```python
from build123d import *

# Parameters (mm, degrees)
BOSS_EXTRUDE1_DEPTH = 2
FILLET1_R           = 2


with BuildPart() as part:
    # Sketch1 → Boss-Extrude1 (new body)
    with BuildSketch(Plane.XY):
        Polygon((0, 0), (13, 0), (13, 1), (9.7, 1), (9.7, 3), (13, 3), (13, 4), (0, 4), (0, 3), (3.3, 3), (3.3, 1), (0, 1), align=None)
    extrude(amount=BOSS_EXTRUDE1_DEPTH)

    # Fillet1
    fillet1_edges = [part.edges().sort_by_distance(p)[0] for p in [
        (6.5, 0, 2),
        (6.5, 4, 2),
    ]]
    fillet(fillet1_edges, radius=FILLET1_R - 0.0001)  # a hair under: the kernel refuses the full size


solid = part.part
```
The listing builds one solid part. Answer for the finished solid, in the listing's coordinates (mm). A direction names the side the tool comes from. Coordinates: 2 decimals unless noted, no trailing zeros. Write each loop counter-clockwise with the first axis right and the second up, starting at its lowest first coordinate (ties: lowest second). Pieces come first, ordered by that corner, then holes. Notation, with made-up numbers: (82.25, 85) -> (135.25, 85) arc R13 ccw to (135.25, 95) -> close; hole circle Ø7 at (61.5, 83.5). An arc over 180 degrees is marked (long way). Write each question's results on one line, items separated by ' | '. Start each with the question number.
1) A cutting plane is placed at D-D (z = 0.8). Determine the outline of the cut face in (x, y), then the cut area to 3 significant figures.
2) Straight lines are drawn through the part: probe 1 along Y at (x, z) = (2.75, 0.7); probe 2 along Y at (x, z) = (12, 1.35); probe 3 along Y at (x, z) = (9, 1.05). For each, find the intervals that lie inside material, in ascending order.
3) For a pull along Y with two mould halves and no side action, classify faces 4 (the flat face through (2, 1, 1)), 5 (the flat face through (13, 3.4, 0.7)), 6 (the cylindrical face through (6.41, 3.65, 1.13)) as +Y half, -Y half, draft (parallel to the pull), parting line (faces both ways), or undercut.
4) Flat-ended cylindrical pins translate along their axes: pin 1 Ø0.5 at (x, z) = (11.5, 0.5) entering from +Y; pin 2 Ø0.5 at (x, z) = (10.5, 1.5) entering from -Y; pin 3 Ø1 at (x, z) = (2.5, 1) entering from +Y. Find the tip coordinate at first contact, or state that the pin passes through.
5) A tool of negligible diameter and unlimited length cuts with its end or side. For faces 1 (the cylindrical face through (6.59, 0.35, 1.13)), 2 (the flat face through (2, 3, 1)), 3 (the flat face through (11, 3, 1)), from which of +Z, -Z, +X, -X, +Y, -Y can it reach the whole face along a straight path? Write none if from no direction.
6) A cutting plane is placed at B-B (z = 1.35). Determine the outline of the cut face in (x, y), then the cut area to 3 significant figures.
Values follow:
1) outline: (0, 0.17) -> (13, 0.17) -> (13, 1) -> (9.7, 1) -> (9.7, 3) -> (13, 3) -> (13, 3.83) -> (0, 3.83) -> (0, 3) -> (3.3, 3) -> (3.3, 1) -> (0, 1) -> close | area: 34.5 mm²
2) probe 1: 0.13 to 1, 3 to 3.87 | probe 2: 0.52 to 1, 3 to 3.48 | probe 3: 0.3 to 3.7
3) face 4: undercut | face 5: draft | face 6: +Y half
4) pin 1: y = 3.98 | pin 2: y = 0.44 | pin 3: y = 3.94
5) face 1: +Z, +X, -X, -Y | face 2: +Z, -Z, -X | face 3: +Z, -Z, +X
6) outline: (0, 0.52) -> (13, 0.52) -> (13, 1) -> (9.7, 1) -> (9.7, 3) -> (13, 3) -> (13, 3.48) -> (0, 3.48) -> (0, 3) -> (3.3, 3) -> (3.3, 1) -> (0, 1) -> close | area: 25.2 mm²
